Geometry: final body of the model. Coordinates: model frame, mm. A direction names the side the tool comes from. Round coordinates to 2 decimals unless told otherwise and drop trailing zeros. Order: outer loops, then holes, each group sorted by start corner. A loop starts at its lowest first (then second) coordinate and runs counter-clockwise, first axis right, second up. Notation, with made-up numbers: M 9,-33.75 L 19,-33.75 A23 ccw 19,-21.75 Z; hole C 27.5,84 d1. An arc over 180 degrees is marked long. Put each result on its own line as item: value. Start each with the question number.
1) Section B-B, the plane x = 28. Return loops of the section in (y, z), then the cut area to 3 significant figures.
2) Section D-D, the plane z = -23. Return loops of the section in (x, y), then the cut area to 3 significant figures.
3) Section C-C, the plane y = 22. Return loops of the section in (x, z).
4) Material intervals for probe 1 along Y at (x, z) = (28, -13); probe 2 along X at (y, z) = (20.5, -15); probe 3 along Y at (x, z) = (43.5, -1.5), sorted ascending. Write a range as [from, to].
5) Access query for faces 1 (the flat face through (31, 10, -25)), 2 (the flat face through (40, 5, -10)), 3 (the flat face through (19, 5, 0)). Directions: +Z, -Z, +X, -X, +Y, -Y. A direction counts if a zero-diameter tool reaches every point of the face in a straight line with its end or side. Return the directions, or none.
6) First-contact query: P1, Ø1.5, axis at x = 32, z = -6.5, coming from the +Y side; P2, Ø2, axis at x = 20, z = -19.5, coming from the +Y side (3 decimals); P3, Ø1.5, axis at x = 6.5, z = -34, coming from the +Y side. Flat tips, straight axial feed; report the tip coordinate or a pass-through.
7) Section A-A, the plane z = -19. Return loops of the section in (x, y).
from build123d import *

# Parameters (mm, degrees)
SKETCH16_W          = 50
SKETCH16_H          = 40
BOSS_EXTRUDE3_DEPTH = 10
CUT_EXTRUDE10_DEPTH = 20
SKETCH21_W          = 20.000334642
SKETCH21_H          = 40
BOSS_EXTRUDE4_DEPTH = 30
CUT_EXTRUDE12_DEPTH = 21


with BuildPart() as part:
    # Sketch16 → Boss-Extrude3 (new body)
    with BuildSketch(Plane(origin=(0, 0, 0), x_dir=(1, 0, 0), z_dir=(0, 1, 0))):
        with Locations((25, 20)):
            Rectangle(SKETCH16_W, SKETCH16_H)
    extrude(amount=BOSS_EXTRUDE3_DEPTH)

    # Sketch20 → Cut-Extrude10 (cut)
    with BuildSketch(Plane.XY):
        Polygon((50, 10), (29.992004992, 10), (50, 0), align=None)
    extrude(amount=-CUT_EXTRUDE10_DEPTH, mode=Mode.SUBTRACT)

    # Sketch21 → Boss-Extrude4 (add)
    with BuildSketch(Plane(origin=(0, 10, 0), x_dir=(1, 0, 0), z_dir=(0, 1, 0))):
        with Locations((10.000167321, 20)):
            Rectangle(SKETCH21_W, SKETCH21_H)
    extrude(amount=BOSS_EXTRUDE4_DEPTH)

    # Sketch22 → Cut-Extrude12 (cut)
    with BuildSketch(Plane(origin=(20.000334642, 0, 0), x_dir=(0, 0, -1), z_dir=(1, 0, 0))):
        Polygon((40, 40), (0, 40), (0, 10), align=None)
    extrude(amount=-CUT_EXTRUDE12_DEPTH, mode=Mode.SUBTRACT)


solid = part.part
Result sheet:
1. outline: M 0,-40 L 10,-40 L 10,0 L 0,0 Z
1. area: 400 mm2
2. outline: M 0,0 L 50,0 L 50,10 L 20,10 L 20,27.25 L 0,27.25 Z
2. area: 845 mm2
3. outline: M 0,-40 L 20,-40 L 20,-16 L 0,-16 Z
4. probe 1: y = [0, 10]
4. probe 2: x = [0, 20]
4. probe 3: y = [0, 3.25]
5. face 1: +Z, -Z, +X, +Y
5. face 2: +Z, +X, +Y
5. face 3: +Z, +X, -X, +Y, -Y
6. P1: stops at y = 9.37
6. P2: stops at y = 25.375
6. P3: stops at y = 36.06
7. outline: M 0,0 L 50,0 L 29.99,10 L 20,10 L 20,24.25 L 0,24.25 Z
